Could you check a few things on this model? Use its own coordinates, in mm. A direction names the side the tool comes from. Give positions to 0.01 mm unless a question says otherwise; leave off trailing zeros. Loops run counter-clockwise (first coordinate to the right, second up) from the corner with the lowest first, then second, coordinate; pieces in that order, holes last. Notation, with made-up numbers: M 8,23.5 L 56,23.5 A20 ccw 56,60.5 Z; hole C -39,21.5 d8. An arc over 180 degrees is marked long. Use a Markdown table: item, result. Add a question column.
1) Suppose I cut it at C-C on y = 79.5. List the corners of the cut face in (x, z) for me, and give its area (3 significant figures).
2) Will these pins go through, and if not, where does the flat tip stop? pin 1 Ø1.5 at (y, z) = (20, 1) entering from -X; pin 2 Ø0.7 at (x, y) = (0, 90.5) entering from +Z; pin 3 Ø1.5 at (y, z) = (23.5, -1.5) entering from -X.
3) Which directions (+Z, -Z, +X, -X, +Y, -Y) give clear straight access to the entire face, cutting with the end or side of a thin tool? Please do faces 1 (the flat face through (0, 6, 1)), 2 (the flat face through (0, 89, 1)), 3 (the cylindrical face through (0, 89.2, -1.5)), 4 (the cylindrical face through (0, 5.7, -1.5)).
4) If I drill on line 1 along X through (y, z) = (31, -1.65); line 2 along Y through (x, z) = (-1.6, -0.45); line 3 along Z through (x, y) = (0.1, 80), over which ranges is the centre line in solid material (lowest first)? Write a range as [from, to].
5) Suppose I cut it at B-B on z = 0. List the corners of the cut face in (x, y) for me.
6) Suppose I cut it at A-A on x = 0. List the corners of the cut face in (y, z) for me.
Autodesk Inventor part; units mm, degrees
ref_plane "YZ Plane" through (0, 0, 0) normal (1, 0, 0) x (0, 1, 0)
ref_plane "XZ Plane" through (0, 0, 0) normal (0, 1, 0) x (-1, 0, 0)
ref_plane "XY Plane" through (0, 0, 0) normal (0, 0, 1) x (1, 0, 0)
sketch "スケッチ1" plane through (0, 0, 0) normal (0, 1, 0) x (-1, 0, 0)
  circle A0 centre (0, 0) radius 2
  dimension "d0" = 4
extrude "押し出し1" add sketch "スケッチ1" along normal blind 97
sketch "スケッチ2" plane through (0, 0, 0) normal (0, -1, 0) x (1, 0, 0)
  circle A0 centre (0, 0) radius 1.5
  line L0 (-1.118, 1) -> (1.118, 1)
  circle A1 centre (0, 0) radius 2
  circle A2 centre (0, 0) radius 2
  dimension "d3" = 3
  dimension "d4" = 1
extrude "押し出し2" cut sketch "スケッチ2" against normal blind 8 contours L0 A0 | A1 picked at (-0.0599, 1.1631)
sketch "スケッチ3" plane through (0, 97, 0) normal (0, 1, 0) x (1, 0, 0)
  arc A0 (1.118, -1) -> (-1.118, -1) centre (0, 0) ccw
  line L0 (1.118, -1) -> (-1.118, -1)
  circle A1 centre (0, 0) radius 2
extrude "押し出し3" cut sketch "スケッチ3" against normal blind 12
sketch "スケッチ4" plane through (0, 97, 0) normal (0, 1, 0) x (1, 0, 0)
  arc A0 (1.118, -1) -> (-1.118, -1) centre (0, 0) ccw
  line L0 (-1.118, -1) -> (1.118, -1)
extrude "押し出し4" cut sketch "スケッチ4" against normal blind 3.7
sketch "スケッチ5" plane through (0, 0, 0) normal (0, -1, 0) x (1, 0, 0)
  line L0 (1.118, 1) -> (-1.118, 1)
  arc A0 (-1.118, 1) -> (1.118, 1) centre (0, 0) ccw
extrude "押し出し5" cut sketch "スケッチ5" against normal blind 3.5
properties part number "screw_screw" material "アルミニウム 6061"
Answer block:
| question | item | result |
|---|---|---|
| 1 | outline | C 0,0 d4 |
| 1 | area | 12.6 mm^2 |
| 2 | pin 1 | stops at x = -1.98 |
| 2 | pin 2 | stops at z = 1 |
| 2 | pin 3 | stops at x = -1.85 |
| 3 | face 1 | +Z, +X, -X, -Y |
| 3 | face 2 | +Z, +X, -X, +Y |
| 3 | face 3 | +Y |
| 3 | face 4 | -Y |
| 4 | line 1 | x = [-1.13, 1.13] |
| 4 | line 2 | y = [8, 85] |
| 4 | line 3 | z = [-2, 2] |
| 5 | outline | M -2,8 L -1.5,8 L -1.5,3.5 L 1.5,3.5 L 1.5,8 L 2,8 L 2,85 L 1.5,85 L 1.5,93.3 L -1.5,93.3 L -1.5,85 L -2,85 Z |
| 6 | outline | M 3.5,-1.5 L 8,-1.5 L 8,-2 L 85,-2 L 85,-1.5 L 93.3,-1.5 L 93.3,1 L 85,1 L 85,2 L 8,2 L 8,1 L 3.5,1 Z |
